The listing builds one solid part. Answer for the finished solid, in the listing's coordinates (mm). Round coordinates to 2 decimals unless told otherwise and drop trailing zeros. Loops run counter-clockwise (first coordinate to the right, second up) from the corner with the lowest first, then second, coordinate; pieces in that order, holes last. Notation, with made-up numbers: M -16.5,32 L -4.5,32 A8 cw -4.5,40 Z; hole C -6,41.5 d6. An arc over 180 degrees is marked long. Answer as a JSON object with one key per item and string values.
Autodesk Inventor part; units mm, degrees
ref_plane "YZ Plane" through (0, 0, 0) normal (1, 0, 0) x (0, 1, 0)
ref_plane "XZ Plane" through (0, 0, 0) normal (0, 1, 0) x (-1, 0, 0)
ref_plane "XY Plane" through (0, 0, 0) normal (0, 0, 1) x (1, 0, 0)
sketch "Sketch1" plane through (0, 0.6434, 0) normal (1, 0, 0) x (0, 1, 0)
  circle A0 centre (15.8, 195.0342) radius 3 construction
  circle A1 centre (15.8, 103.0342) radius 3 construction
  circle A2 centre (20.0554, 146.9079) radius 1.45 construction
  circle A3 centre (-24.7132, 132.4283) radius 3.5 construction
  circle A4 centre (-24.9297, 123.6553) radius 3.5 construction
  circle A5 centre (15.1664, 127.0554) radius 4 construction
  circle A6 centre (-25.4429, 102.8495) radius 4 construction
  circle A7 centre (-24.2, 153.2342) radius 4 construction
  circle A8 centre (14.5499, 102.063) radius 2.95 construction
  circle A9 centre (16.8187, 194.035) radius 2.95 construction
  line L0 (-1.4549, 93.9552) -> (-1.2206, 103.4531) construction
  line L1 (-1.4549, 93.9552) -> (16.1397, 93.5212) construction
  arc A10 (16.1397, 93.5212) -> (21.2615, 98.3964) centre (16.263, 98.5197) ccw construction
  line L2 (21.2615, 98.3964) -> (23.652, 195.301) construction
  arc A11 (23.652, 195.301) -> (18.7768, 200.4228) centre (18.6535, 195.4243) ccw construction
  line L3 (18.7768, 200.4228) -> (12.8677, 200.5685) construction
  arc A12 (12.8677, 200.5685) -> (8.4173, 198.0753) centre (12.7444, 195.57) ccw construction
  line L4 (8.4173, 198.0753) -> (0.9275, 185.1387) construction
  line L5 (0.1833, 154.9709) -> (0.9275, 185.1387) construction
  line L6 (-7.9473, 155.1714) -> (0.1833, 154.9709) construction
  line L7 (-7.8733, 158.1705) -> (-7.9473, 155.1714) construction
  line L8 (-2.3058, 158.0332) -> (-7.8733, 158.1705) construction
  line L9 (-1.7513, 180.5119) -> (-2.3058, 158.0332) construction
  line L10 (-1.7513, 180.5119) -> (-12.8987, 161.2579) construction
  line L11 (-29.7936, 161.6747) -> (-12.8987, 161.2579) construction
  arc A13 (-29.7936, 161.6747) -> (-31.8423, 159.7246) centre (-29.8429, 159.6753) ccw construction
  line L12 (-31.8423, 159.7246) -> (-33.3959, 96.7438) construction
  arc A14 (-33.3959, 96.7438) -> (-31.4458, 94.695) centre (-31.3965, 96.6944) ccw construction
  line L13 (-31.4458, 94.695) -> (-3.885, 94.0152) construction
  line L14 (-3.7247, 100.514) -> (-3.885, 94.0152) construction
  line L15 (-9.2922, 100.6513) -> (-3.7247, 100.514) construction
  line L16 (-9.2182, 103.6504) -> (-9.2922, 100.6513) construction
  line L17 (-1.2206, 103.4531) -> (-9.2182, 103.6504) construction
  circle A15 centre (14.1273, 157.9245) radius 4.7908 construction
  line L18 (17.6, 201.4682) -> (11.6, 201.4682)
  line L19 (6.6, 196.4682) -> (6.6, 99.5342)
  line L20 (11.6, 94.5342) -> (17.6, 94.5342)
  line L21 (22.6, 99.5342) -> (22.6, 196.4682)
  arc A16 (11.6, 201.4682) -> (6.6, 196.4682) centre (11.6, 196.4682) ccw
  arc A17 (22.6, 196.4682) -> (17.6, 201.4682) centre (17.6, 196.4682) ccw
  arc A18 (17.6, 94.5342) -> (22.6, 99.5342) centre (17.6, 99.5342) ccw
  arc A19 (6.6, 99.5342) -> (11.6, 94.5342) centre (11.6, 99.5342) ccw
  circle A20 centre (20.0554, 146.9079) radius 1.45
  circle A21 centre (15.8, 103.0342) radius 3
  circle A22 centre (15.8, 195.0342) radius 3
  circle A23 centre (20.198, 175.9006) radius 1.45
  circle A24 centre (20.198, 127.1464) radius 1.45
  point P0 (-0.6434, 0)
  point P1 (6.6, 94.5342)
  dimension "d0" = 16
  dimension "d1" = 5
  dimension "d2" = 2.9
  dimension "d3" = 2.9
extrude "Extrusion1" add sketch "Sketch1" along normal blind 10
properties part number "Neje_Base_Slide_y_stop"
Item 1: Flat-ended cylindrical pins translate along their axes: P1, Ø3.5, axis at y = 16.44, z = 103.03, coming from the +X side; P2, Ø1, axis at x = 6.5, y = 21, coming from the +Z side. Find the tip coordinate at first contact, or state that the pin passes through.
Values follow:
{"P1": "through", "P2": "z = 200.93"}
Item 2: Straight lines are drawn through the part: line 1 (Z direction, x = 2.75, y = 13.75); line 2 (Z direction, x = 9.5, y = 19); line 3 (Y direction, x = 7.25, z = 195). For each, find the intervals that lie inside material, in ascending order.
Values follow:
{"line 1": "94.53 to 101.71, 104.36 to 193.71, 196.36 to 201.47", "line 2": "94.59 to 101.46, 104.6 to 193.46, 196.6 to 201.41", "line 3": "7.24 to 13.44, 19.44 to 23.24"}
Item 3: Determine the mould class of faces 1 (the face through (4.93, 8.669, 199.965)), 2 (the face through (4.93, 20.527, 128.562)), 3 (the face through (5, 15, 94.534)) for opening direction Z: released by +Z, released by -Z, zero draft, split by the parting line, or undercut.
Values follow:
{"face 1": "released by +Z", "face 2": "undercut", "face 3": "released by -Z"}
Item 4: The part is cut by section A-A (x = 5.75). Give the vertices of the cut face in (y, z), then the cut area to 3 significant figures.
Values follow:
{"outline": "M 7.24,99.53 A5 ccw 12.24,94.53 L 18.24,94.53 A5 ccw 23.24,99.53 L 23.24,196.47 A5 ccw 18.24,201.47 L 12.24,201.47 A5 ccw 7.24,196.47 Z; hole C 16.44,103.03 d6; hole C 16.44,195.03 d6; hole C 20.7,146.91 d2.9; hole C 20.84,127.15 d2.9; hole C 20.84,175.9 d2.9", "area": "1,610 mm^2"}
Item 5: The part is cut by section B-B (z = 104). Give the vertices of the cut face in (x, y).
Values follow:
{"outline": "M 0,7.24 L 10,7.24 L 10,13.6 L 0,13.6 Z; M 0,19.28 L 10,19.28 L 10,23.24 L 0,23.24 Z"}
